Autodesk Inventor part; units mm, degrees
ref_plane "YZ Plane" through (0, 0, 0) normal (1, 0, 0) x (0, 1, 0)
ref_plane "XZ Plane" through (0, 0, 0) normal (0, 1, 0) x (-1, 0, 0)
ref_plane "XY Plane" through (0, 0, 0) normal (0, 0, 1) x (1, 0, 0)
sketch "BasePlate" plane through (0, 0, 0) normal (0, 0, 1) x (1, 0, 0)
  line L0 (56.5, 56.5) -> (0, 56.5)
  line L1 (0, 56.5) -> (0, 0)
  line L2 (0, 0) -> (56.5, 0)
  line L3 (56.5, 0) -> (56.5, 56.5)
  line L4 (96.5, 96.5) -> (-40, 96.5)
  line L5 (-40, 96.5) -> (-40, -40)
  line L6 (-40, -40) -> (96.5, -40)
  line L7 (96.5, -40) -> (96.5, 96.5)
  circle A0 centre (-4, 60.5) radius 1.75
  circle A1 centre (-4, 60.5) radius 5.25
  circle A2 centre (60.5, 60.5) radius 5.25
  circle A3 centre (60.5, 60.5) radius 1.75
  circle A4 centre (-4, -4) radius 5.25
  circle A5 centre (-4, -4) radius 1.75
  circle A6 centre (60.5, -4) radius 5.25
  circle A7 centre (60.5, -4) radius 1.75
  line L8 (58.5, 58.5) -> (-2, 58.5)
  line L9 (-2, 58.5) -> (-2, -2)
  line L10 (-2, -2) -> (58.5, -2)
  line L11 (58.5, -2) -> (58.5, 58.5)
  line L12 (56.5, 38.5) -> (58.5, 38.5)
  line L13 (56.5, 18) -> (58.5, 18)
  circle A8 centre (-32, 88.5) radius 4.5
  circle A9 centre (87.5, 88.5) radius 4.5
  circle A10 centre (-32, -31) radius 4.5
  circle A11 centre (87.5, -31) radius 4.5
  line L14 (-40, 61.5) -> (-9.1539, 61.5)
  line L15 (-9.1539, 61.5) -> (-9.1539, 59.5)
  line L16 (-9.1539, 59.5) -> (-40, 59.5)
  line L17 (-40, 59.5) -> (-40, 61.5)
  line L18 (-3, 96.5) -> (-3, 65.6539)
  line L19 (-5, 65.6539) -> (-5, 96.5)
  line L20 (-5, 96.5) -> (-3, 96.5)
  line L21 (-3, 65.6539) -> (-5, 65.6539)
  line L22 (0, 56.5) -> (56.5, 0)
  line L23 (56.5, 56.5) -> (0, 0)
  line L24 (-9.1539, -3) -> (-9.1539, -5)
  line L25 (-40, -5) -> (-40, -3)
  line L26 (-9.1539, -5) -> (-40, -5)
  line L27 (-40, -3) -> (-9.1539, -3)
  line L28 (-3, -9.1539) -> (-3, -40)
  line L29 (-5, -40) -> (-5, -9.1539)
  line L30 (-3, -40) -> (-5, -40)
  line L31 (-5, -9.1539) -> (-3, -9.1539)
  line L32 (59.5, -9.1539) -> (61.5, -9.1539)
  line L33 (61.5, -40) -> (59.5, -40)
  line L34 (61.5, -9.1539) -> (61.5, -40)
  line L35 (59.5, -40) -> (59.5, -9.1539)
  line L36 (65.6539, -3) -> (96.5, -3)
  line L37 (96.5, -5) -> (65.6539, -5)
  line L38 (96.5, -3) -> (96.5, -5)
  line L39 (65.6539, -5) -> (65.6539, -3)
  line L40 (65.6539, 59.5) -> (65.6539, 61.5)
  line L41 (96.5, 61.5) -> (96.5, 59.5)
  line L42 (65.6539, 61.5) -> (96.5, 61.5)
  line L43 (96.5, 59.5) -> (65.6539, 59.5)
  line L44 (59.5, 65.6539) -> (59.5, 96.5)
  line L45 (61.5, 96.5) -> (61.5, 65.6539)
  line L46 (59.5, 96.5) -> (61.5, 96.5)
  line L47 (61.5, 65.6539) -> (59.5, 65.6539)
  point P0 (28.25, 28.25)
  dimension "d0" = 56.5
  dimension "d102" = 40
  dimension "d104" = 3.5
  dimension "d105" = 3.5
  dimension "d106" = 4
  dimension "d107" = 4
  dimension "d110" = 64.5
  dimension "d113" = 64.5
  dimension "d116" = 2
  dimension "d117" = 20
  dimension "d118" = 20
  dimension "d119" = 9
  dimension "d120" = 8
  dimension "d121" = 8
  dimension "d124" = 119.5
  dimension "d127" = 119.5
  dimension "d130" = 2
  dimension "d133" = 90
  dimension "d137" = 360
extrude "Extrusion8" add sketch "BasePlate" along normal blind 5 contours L23 L22 L0 | L0 L1 L2 L3 L13 L11 A6 L10 A4 L9 A1 L8 A2 L12 | L3 L22 L23 | L22 L23 L1 | L12 L11 L13 L3 | L22 L2 L23 | L11 A2 L43 L7 L36 A6 | L11 L8 A2 L47 L40 | A2 L8 L11 | L11 L10 A6 | A6 L39 L32 L10 L11 | L8 A1 L18 L4 L44 A2 | L40 A2 | A2 L42 L7 L43 | L36 L7 L37 A6 | A6 L39 | A6 L35 L6 L28 A4 L10 | L44 L4 L45 A2 | A2 L47 | L8 L9 A1 L15 L21 | A1 L9 L8 | A2 L45 L4 L7 L42 | L37 L7 L6 L34 A6 | L32 A6 | A6 L34 L6 L35 | L10 L9 A4 | A4 L31 L24 L9 L10 | L9 A4 L27 L5 L16 A1 | L18 A1 L19 L4 | L16 L5 L14 A1 | A1 L15 | L21 A1 | L6 L29 A4 L28 | A4 L31 | L24 A4 | A4 L26 L5 L27 | L19 A1 L14 L5 L4 | L6 L5 L26 A4 L29 | A0 | A3 | A5 | A7
extrude "Extrusion9" add sketch "BasePlate" along normal blind 56.1 contours L0 L1 L2 L3 L13 L11 A6 L10 A4 L9 A1 L8 A2 L12 | L11 L8 A2 L47 L40 | A2 L8 L11 | L11 L10 A6 | A6 L39 L32 L10 L11 | L40 A2 | A2 L42 L7 L43 | L36 L7 L37 A6 | A6 L39 | L44 L4 L45 A2 | A2 L47 | L8 L9 A1 L15 L21 | A1 L9 L8 | L32 A6 | A6 L34 L6 L35 | L10 L9 A4 | A4 L31 L24 L9 L10 | L18 A1 L19 L4 | L16 L5 L14 A1 | A1 L15 | L21 A1 | L6 L29 A4 L28 | A4 L31 | L24 A4 | A4 L26 L5 L27
chamfer "Chamfer3" distance 10 angle 45 2 edges at (57.5, 18, 56.1) (57.5, 38.5, 56.1)
chamfer "Chamfer4" distance 30 angle 45 8 edges at (96.5, -4, 56.1) (60.5, -40, 56.1) (-4, -40, 56.1) (-40, -4, 56.1) (-40, 60.5, 56.1) (-4, 96.5, 56.1) (60.5, 96.5, 56.1) (96.5, 60.5, 56.1)
fillet "Fillet3" radius 9 4 edges at (96.5, -40, 2.5) (96.5, 96.5, 2.5) (-40, 96.5, 2.5) (-40, -40, 2.5)
properties part number "TurntableStand"
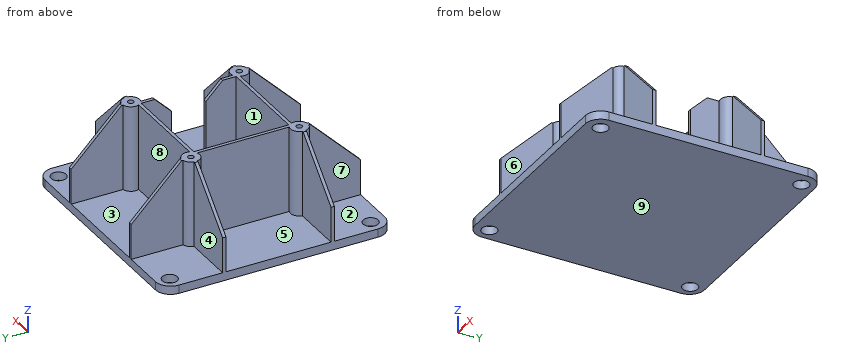
Design review of the part built by this model. Coordinates are the model's own, in mm. Face numbers are marked on the shaded views. A direction names the side the tool comes from. Give positions to 0.01 mm unless a question says otherwise; leave off trailing zeros. Write each loop counter-clockwise with the first axis right and the second up, starting at its lowest first coordinate (ties: lowest second). Pieces come first, ordered by that corner, then holes. Notation, with made-up numbers: M 45.25,-38.75 L 87.25,-38.75 A18 ccw 87.25,-30.75 Z; hole C 34,49 d8. An arc over 180 degrees is marked long. Return JSON: item names as keys, results as strings. Group by question number.
Item 1: The part is to be moulded in two halves that separate along X. For the marked faces 6, 7, 8 and 9, say which applies: pulls with the +X half, pulls with the -X half, needs draft (parallel to the pull), parting line crosses it, or undercut.
Item 2: Take a section at C-C (z = 28.5). Count the separate pieces of the cut face and the enclosed holes in it, plus the area to 3 significant figures.
Item 3: Clearance check with flat-ended pins moving along their axes: pin 1 Ø2 at (x, z) = (57.5, 17.5) entering from -Y; pin 2 Ø9.5 at (x, z) = (-29, 38.5) entering from -Y; pin 3 Ø15.5 at (x, z) = (31.5, 42) entering from +Y. State where each tip first meets the part, or that it passes through.
Item 4: Take a section at A-A (x = 76). Give the boundary of the cut face in (y, z), plus the area to 3 significant figures.
Item 5: Take a section at B-B (y = 45.5). Give the boundary of the cut face in (x, z), plus the area to 3 significant figures.
Item 6: Tool access review of the marked faces 1, 2, 3, 4 and 5: name each direction out of +Z, -Z, +X, -X, +Y, -Y from which nothing blocks a thin tool from reaching the whole face with its end or side.
Item 7: Wall thickness on line 1 along X through (y, z) = (-4, 24); line 2 along Y through (x, z) = (87, 1); line 3 along X through (y, z) = (67, 15.5): over which ranges is each line inside the solid? List them lowest first.
Return value:
{
 "1": {"face 6": "undercut", "face 7": "pulls with the -X half", "face 8": "undercut", "face 9": "needs draft"},
 "2": {"separate pieces": "1", "enclosed holes": "4", "area": "1,170 mm2"},
 "3": {"pin 1": "stops at y = -8.85", "pin 2": "stops at y = -5", "pin 3": "stops at y = 58.5"},
 "4": {"outline": "M -40,0 L 96.5,0 L 96.5,5 L 61.5,5 L 61.5,46.6 L 59.5,46.6 L 59.5,5 L -3,5 L -3,46.6 L -5,46.6 L -5,5 L -40,5 Z", "area": "849 mm2"},
 "5": {"outline": "M -40,0 L 96.5,0 L 96.5,5 L 58.5,5 L 58.5,53.1 L 56.5,53.1 L 56.5,5 L 0,5 L 0,56.1 L -2,56.1 L -2,5 L -40,5 Z", "area": "881 mm2"},
 "6": {"face 1": "+Z", "face 2": "+Z, -X, -Y", "face 3": "+Z, +Y", "face 4": "+Z, -X, +Y", "face 5": "+Z, -X"},
 "7": {"line 1": "x = -40 to -5.75, -2.25 to 1.25, 55.25 to 58.75, 62.25 to 96.5", "line 2": "y = -40 to -35.47, -26.53 to 84.03, 92.97 to 96.5", "line 3": "x = -5 to -3, 59.5 to 61.5"}
}
